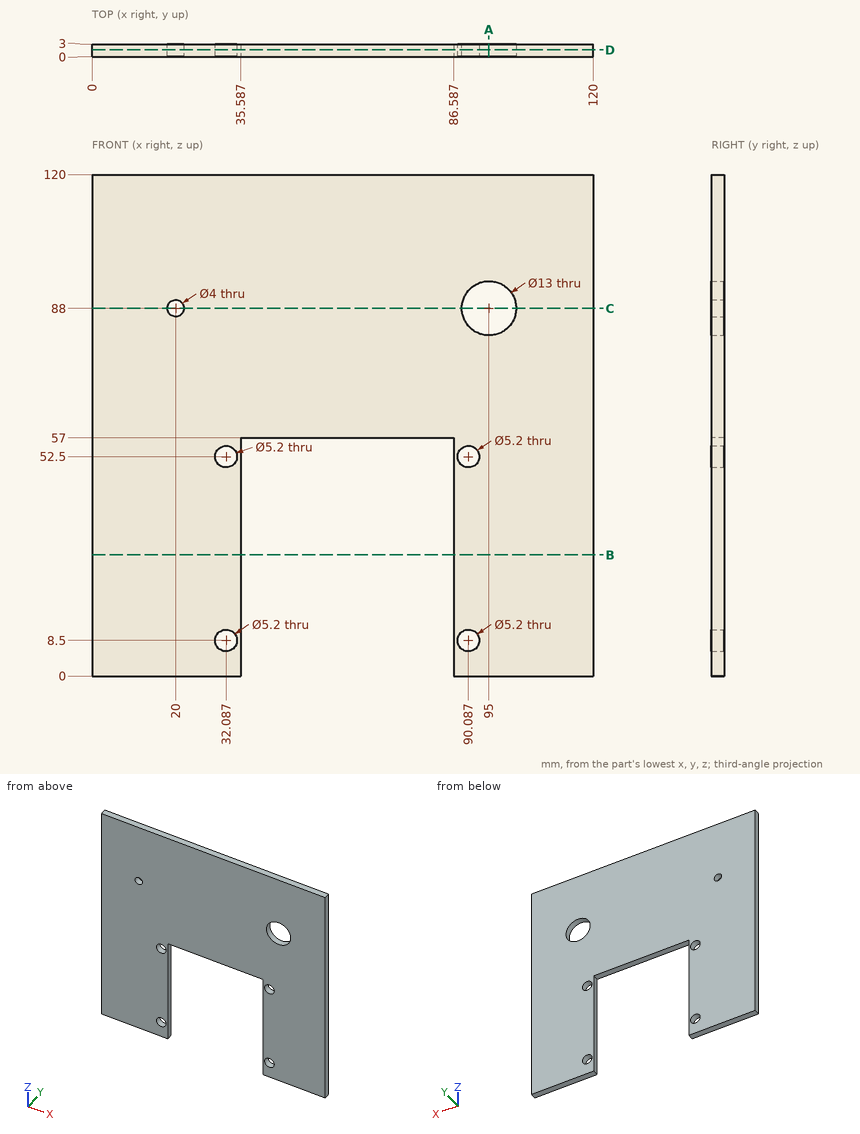
Source: three-view drawing plus pictorial views. Frame: mm from the lowest corner of the part. Round coordinates to 2 decimals unless told otherwise and drop trailing zeros. Loops run counter-clockwise (first coordinate to the right, second up) from the corner with the lowest first, then second, coordinate; pieces in that order, holes last.
Q1. Section D-D on y = 1.6. Return loops of the section in (x, z).
Q2. Section B-B on z = 29. Return loops of the section in (x, y), plus the area to 3 significant figures.
Q3. Material intervals for L1, parallel to X at y = 1.05, z = 52.5; L2, parallel to X at y = 1.75, z = 88; L3, parallel to Z at x = 95, y = 1.9, sorted ascending.
Q4. Section A-A on x = 95. Return loops of the section in (y, z).
Q5. Section C-C on z = 88. Return loops of the section in (x, y), plus the area to 3 significant figures.
Evaluation:
1. outline: (0, 0) - (35.59, 0) - (35.59, 57) - (86.59, 57) - (86.59, 0) - (120, 0) - (120, 120) - (0, 120) - close; hole circle Ø4 at (20, 88); hole circle Ø5.2 at (32.09, 8.5); hole circle Ø5.2 at (32.09, 52.5); hole circle Ø5.2 at (90.09, 8.5); hole circle Ø5.2 at (90.09, 52.5); hole circle Ø13 at (95, 88)
2. outline: (0, 0) - (35.59, 0) - (35.59, 3) - (0, 3) - close; (86.59, 0) - (120, 0) - (120, 3) - (86.59, 3) - close
2. area: 207 mm2
3. L1: x = 0 to 29.49, 34.69 to 35.59, 86.59 to 87.49, 92.69 to 120
3. L2: x = 0 to 18, 22 to 88.5, 101.5 to 120
3. L3: z = 0 to 81.5, 94.5 to 120
4. outline: (0, 0) - (3, 0) - (3, 81.5) - (0, 81.5) - close; (0, 94.5) - (3, 94.5) - (3, 120) - (0, 120) - close
5. outline: (0, 0) - (18, 0) - (18, 3) - (0, 3) - close; (22, 0) - (88.5, 0) - (88.5, 3) - (22, 3) - close; (101.5, 0) - (120, 0) - (120, 3) - (101.5, 3) - close
5. area: 309 mm2
